Could you check a few things on this model? Use its own coordinates, in mm. A direction names the side the tool comes from. Give positions to 0.01 mm unless a question says otherwise; leave off trailing zeros. Loops run counter-clockwise (first coordinate to the right, second up) from the corner with the lowest first, then second, coordinate; pieces in that order, holes last. Notation, with made-up numbers: M 86,-25 L 102,-25 A22 cw 102,2 Z; hole C 79.5,84.5 d8. An arc over 180 degrees is marked long. Use a Markdown table: item, result. Add a question column.
1) We'd pull the mould along X, two halves only. Please class faces 1 (the flat face through (-2.153, 2, -49)), 2 (the cylindrical face through (-68.401, 1.61, -68.322)), 3 (the flat face through (-1, 3.175, -1)): +X half, -X half, draft (parallel to the pull), parting line (faces both ways), or undercut.
2) Suppose I cut it at B-B on y = 0.65. Count the separate pieces of the cut face and the enclosed holes in it, and give its area (3 significant figures).
3) Which directions (+Z, -Z, +X, -X, +Y, -Y) give clear straight access to the entire face, cutting with the end or side of a thin tool? Please do faces 4 (the cylindrical face through (0.047, 1.61, -53.846)), 5 (the flat face through (7.383, 2, -56)), 6 (the flat face through (-30, 2, -69.85)).
4) Suppose I cut it at A-A on x = 26.67. List the corners of the cut face in (y, z) for me (3 decimals).
5) If I drill on line 1 along Z through (x, y) = (0, 2.1); line 2 along X through (y, z) = (1.2, 63); line 3 along X through (y, z) = (3, -59), over which ranges is the centre line in solid material (lowest first)? Write a range as [from, to].
6) Will this pin go through, and if not, where does the flat tip stop? pin 1 Ø1 at (x, y) = (17, 1.5) entering from -Z.
```python
from build123d import *

# Parameters (mm, degrees)
SKETCH1_W           = 139.7
SKETCH1_H           = 139.7
SKETCH1_R           = 2.4892
BOSS_EXTRUDE1_DEPTH = 3.175
SKETCH2_W           = 10.16
SKETCH2_H           = 24.13
CUT_EXTRUDE2_DEPTH  = 3.175
SKETCH3_R           = 6.35
SKETCH3_R_2         = 1.905
CUT_EXTRUDE4_DEPTH  = 3.175
FILLET2_R           = 5.08
FILLET3_R           = 5.08
FILLET4_R           = 5.08
FILLET5_R           = 5.08
FILLET6_R           = 2.54
FILLET8_R           = 2.54


with BuildPart() as part:
    # Sketch1 → Boss-Extrude1 (new body)
    with BuildSketch(Plane(origin=(0, 0, 0), x_dir=(1, 0, 0), z_dir=(0, 1, 0))):
        Rectangle(SKETCH1_W, SKETCH1_H)
        with Locations(Location((62.484, -62.484, 0), (0, 0, 270))):
            Circle(SKETCH1_R, mode=Mode.SUBTRACT)
        with Locations(Location((-62.484, 62.484, 0), (0, 0, 270))):
            Circle(SKETCH1_R, mode=Mode.SUBTRACT)
        with Locations(Location((62.484, 62.484, 0), (0, 0, 270))):
            Circle(SKETCH1_R, mode=Mode.SUBTRACT)
        with Locations(Location((-62.484, -62.484, 0), (0, 0, 270))):
            Circle(SKETCH1_R, mode=Mode.SUBTRACT)
    extrude(amount=BOSS_EXTRUDE1_DEPTH)

    # Sketch2 → Cut-Extrude2 (cut)
    with BuildSketch(Plane(origin=(0, 3.175, 0), x_dir=(1, 0, 0), z_dir=(0, 1, 0))):
        with Locations((12.46265, 57.785)):
            Rectangle(SKETCH2_W, SKETCH2_H)
        with BuildLine():
            ThreePointArc((-2.15265, 45.344), (0, 43.19135), (2.15265, 45.344))
            Line((2.15265, 45.344), (2.15265, 51.694))
            ThreePointArc((2.15265, 51.694), (0, 53.84665), (-2.15265, 51.694))
            Line((-2.15265, 51.694), (-2.15265, 45.344))
        make_face()
        with BuildLine():
            ThreePointArc((2.15265, 17.658), (0, 19.81065), (-2.15265, 17.658))
            Line((-2.15265, 17.658), (-2.15265, 11.308))
            ThreePointArc((-2.15265, 11.308), (0, 9.15535), (2.15265, 11.308))
            Line((2.15265, 11.308), (2.15265, 17.658))
        make_face()
    extrude(amount=-CUT_EXTRUDE2_DEPTH, mode=Mode.SUBTRACT)

    # Sketch3 → Cut-Extrude4 (cut)
    with BuildSketch(Plane(origin=(0, 3.175, 0), x_dir=(1, 0, 0), z_dir=(0, 1, 0))):
        with Locations(Location((0.254, -46.198145278, 0), (0, 0, 270))):
            Circle(SKETCH3_R)
        with Locations(Location((26.67, -46.198145278, 0), (0, 0, 270))):
            Circle(SKETCH3_R_2)
        with Locations(Location((-14.224, -46.198145278, 0), (0, 0, 270))):
            Circle(SKETCH3_R_2)
    extrude(amount=-CUT_EXTRUDE4_DEPTH, mode=Mode.SUBTRACT)

    # Fillet2
    fillet2_edges = [part.edges().sort_by_distance(p)[0] for p in [
        (-69.85, 1.5875, 69.85),
    ]]
    fillet(fillet2_edges, radius=FILLET2_R)

    # Fillet3
    fillet3_edges = [part.edges().sort_by_distance(p)[0] for p in [
        (69.85, 1.5875, 69.85),
    ]]
    fillet(fillet3_edges, radius=FILLET3_R)

    # Fillet4
    fillet4_edges = [part.edges().sort_by_distance(p)[0] for p in [
        (69.85, 1.5875, -69.85),
    ]]
    fillet(fillet4_edges, radius=FILLET4_R)

    # Fillet5
    fillet5_edges = [part.edges().sort_by_distance(p)[0] for p in [
        (-69.85, 1.5875, -69.85),
    ]]
    fillet(fillet5_edges, radius=FILLET5_R)

    # Fillet6
    fillet6_edges = [part.edges().sort_by_distance(p)[0] for p in [
        (7.38265, 1.5875, -69.85),
    ]]
    fillet(fillet6_edges, radius=FILLET6_R)

    # Fillet8
    fillet8_edges = [part.edges().sort_by_distance(p)[0] for p in [
        (17.54265, 1.5875, -69.85),
    ]]
    fillet(fillet8_edges, radius=FILLET8_R)


solid = part.part
```
Answer block:
| question | item | result |
|---|---|---|
| 1 | face 1 | undercut |
| 1 | face 2 | -X half |
| 1 | face 3 | draft |
| 2 | separate pieces | 1 |
| 2 | enclosed holes | 9 |
| 2 | area | 18,900 mm^2 |
| 3 | face 4 | +Y, -Y |
| 3 | face 5 | -Z, +Y, -Y |
| 3 | face 6 | -Z, +X, -X, +Y, -Y |
| 4 | outline | M 0,-69.85 L 3.175,-69.85 L 3.175,44.293 L 0,44.293 Z; M 0,48.103 L 3.175,48.103 L 3.175,69.85 L 0,69.85 Z |
| 5 | line 1 | z = [-69.85, -53.85], [-43.19, -19.81], [-9.16, 39.85], [52.54, 69.85] |
| 5 | line 2 | x = [-69.85, -64.92], [-60.05, 60.05], [64.92, 69.85] |
| 5 | line 3 | x = [-69.85, 7.38], [17.54, 69.85] |
| 6 | pin 1 | stops at z = -45.72 |
